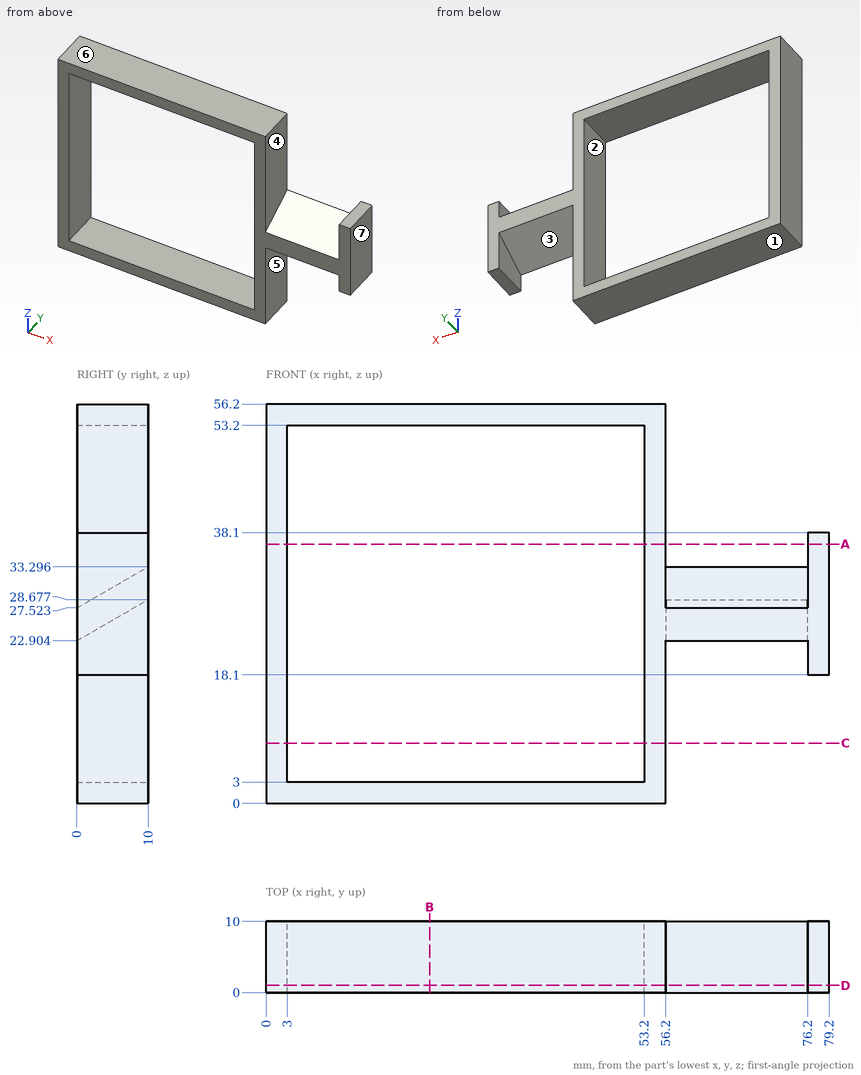
Geometry: see drawing. Coordinates: mm, zero at the bounding-box minimum. A direction names the side the tool comes from. Coordinates: 2 decimals unless noted, no trailing zeros. Order: outer loops, then holes, each group sorted by start corner. A loop starts at its lowest first (then second) coordinate and runs counter-clockwise, first axis right, second up. Notation, with made-up numbers: (-32.5, 31.25) - (15.5, 31.25) arc R25 cw to (15.5, 57.25) - close; hole circle Ø7 at (-4.75, 64). An arc over 180 degrees is marked (long way). Write each question's results on one line, items separated by ' | '.
1) Line query: line 1 (X direction, y = 5.75, z = 31.5); line 2 (X direction, y = 9, z = 51.5). Output: solid intervals per line, ascending. Write a range as from..to.
Results list:
line 1: 0..3, 53.2..56.2, 76.2..79.2 | line 2: 0..3, 53.2..56.2
2) Pin query (flat end, axial travel): pin 1 (5 mm diameter, centred on y = 4, z = 9.5, fed in from +X); pin 2 (0.9 mm diameter, centred on x = 78, y = 4.5, fed in from +Z); pin 3 (1.5 mm diameter, centred on x = 77.5, y = 4.5, fed in from -Z). Return the tip coordinate at first contact, or that it passes through.
Results list:
pin 1: x = 56.2 | pin 2: z = 38.1 | pin 3: z = 18.1
3) Set-up query: the marked faces 1, 2, 3 and 4. Return all of +Z, -Z, +X, -X, +Y, -Y with unobstructed straight access to the full face (end or side cutting, diameter ignored); none if empty.
Results list:
face 1: -Z, +X, -X, +Y, -Y | face 2: +Y, -Y | face 3: -Z, +Y | face 4: +Z, -Y
4) Section B-B, the plane x = 23. Return loops of the section in (y, z).
Results list:
outline: (0, 0) - (10, 0) - (10, 3) - (0, 3) - close; (0, 53.2) - (10, 53.2) - (10, 56.2) - (0, 56.2) - close
5) Pull-direction query (X, two-part tool) for the marked faces 5, 6 and 7; classes: pulls with the +X half, pulls with the -X half, needs draft (parallel to the pull), parting line crosses it, or undercut.
Results list:
face 5: undercut | face 6: needs draft | face 7: pulls with the +X half
6) Section A-A, the plane z = 36.5. Return loops of the section in (x, y).
Results list:
outline: (0, 0) - (3, 0) - (3, 10) - (0, 10) - close; (53.2, 0) - (56.2, 0) - (56.2, 10) - (53.2, 10) - close; (76.2, 0) - (79.2, 0) - (79.2, 10) - (76.2, 10) - close
7) Section D-D, the plane y = 1. Return loops of the section in (x, z).
Results list:
outline: (0, 0) - (56.2, 0) - (56.2, 23.48) - (76.2, 23.48) - (76.2, 18.1) - (79.2, 18.1) - (79.2, 38.1) - (76.2, 38.1) - (76.2, 28.1) - (56.2, 28.1) - (56.2, 56.2) - (0, 56.2) - close; hole (3, 3) - (53.2, 3) - (53.2, 53.2) - (3, 53.2) - close
8) Section C-C, the plane z = 8.5. Return loops of the section in (x, y).
Results list:
outline: (0, 0) - (3, 0) - (3, 10) - (0, 10) - close; (53.2, 0) - (56.2, 0) - (56.2, 10) - (53.2, 10) - close
